```python
from build123d import *

# Parameters (mm, degrees)
F0_R      = 12.7
F1_DEPTH  = 76.2
F3_R      = 17.5641
F4_DEPTH  = 10.16
F6_DEPTH  = 8.636
F7_R      = 12.7
F8_DEPTH  = 76.2
F9_R      = 17.5641
F10_DEPTH = 10.16


with BuildPart() as f1:
    # F0 (on Top) → F1 (new body)
    with BuildSketch(Plane.XY):
        Circle(F0_R)
    extrude(amount=F1_DEPTH)

    # F3 (on offset) → F4 (join)
    with BuildSketch(Plane.XY.offset(74.422)):
        Circle(F3_R)
    extrude(amount=F4_DEPTH)

    # F5 (on Top) → F6 (join)
    with BuildSketch(Plane.XY):
        Polygon((-21.659788, 21.301638), (-21.659788, -20.368967), (60.890212, -20.368967), (60.890212, 0), (60.890212, 21.301638), align=None)
        Polygon((60.890212, 0), (60.890212, -20.368967), (143.440212, -20.368967), (143.440212, 21.301638), (60.890212, 21.301638), align=None)
    extrude(amount=-F6_DEPTH)

    # F7 (on face) → F8 (join)
    with BuildSketch(Plane.XY):
        with Locations((60.890212, 0)):
            Circle(F7_R)
        with Locations((121.774012, 0)):
            Circle(F7_R)
    extrude(amount=F8_DEPTH)

    # F9 (on offset) → F10 (join)
    with BuildSketch(Plane.XY.offset(74.422)):
        with Locations((60.890212, 0)):
            Circle(F9_R)
        with Locations((121.774012, 0)):
            Circle(F9_R)
    extrude(amount=F10_DEPTH)


solid = f1.part
```
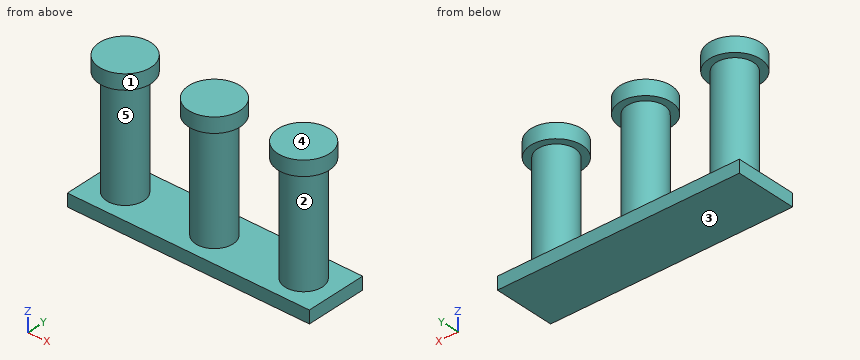
Geometry: final body of the model. Coordinates: model frame, mm. Face numbers are marked on the shaded views. A direction names the side the tool comes from. Round coordinates to 2 decimals unless told otherwise and drop trailing zeros. Write each loop counter-clockwise with the first axis right and the second up, starting at its lowest first coordinate (ties: lowest second). Pieces come first, ordered by that corner, then holes.
Item 1: Section query D-D (y = 0). Return loops of the section in (x, z).
Item 2: Set-up query: the marked faces 1, 2 and 3. Return all of +Z, -Z, +X, -X, +Y, -Y with unobstructed straight access to the full face (end or side cutting, diameter ignored); none if empty.
Item 3: Material intervals for L1, parallel to X at y = 0.5, z = 31; L2, parallel to X at y = 9, z = 17.5; L3, parallel to Z at x = 13, y = -2, sorted ascending.
Item 4: Mould query, pull axis X, two halves, no side actions, for the marked faces 4 and 5. Classes: +X half, -X half, draft (parallel to the pull), parting line (faces both ways), or undercut.
Item 5: Section query B-B (x = 0). Return loops of the section in (y, z).
Item 6: Pin query (flat end, axial travel): P1, Ø12, axis at x = 72.5, z = 40.5, coming from the -Y side; P2, Ø1.5, axis at x = 53, z = 49.5, coming from the +Y side; P3, Ø8, axis at x = 66, z = 64, coming from the -Y side. Return the tip coordinate at first contact, or that it passes through.
Item 7: Section query A-A (y = -16). Return loops of the section in (x, z), plus the area to 3 significant figures.
Item 8: Section query C-C (z = 76.5). Return loops of the section in (x, y), plus the area to 3 significant figures.
Completed:
1. outline: (-21.66, -8.64) - (143.44, -8.64) - (143.44, 0) - (134.47, 0) - (134.47, 74.42) - (139.34, 74.42) - (139.34, 84.58) - (104.21, 84.58) - (104.21, 74.42) - (109.07, 74.42) - (109.07, 0) - (73.59, 0) - (73.59, 74.42) - (78.45, 74.42) - (78.45, 84.58) - (43.33, 84.58) - (43.33, 74.42) - (48.19, 74.42) - (48.19, 0) - (12.7, 0) - (12.7, 74.42) - (17.56, 74.42) - (17.56, 84.58) - (-17.56, 84.58) - (-17.56, 74.42) - (-12.7, 74.42) - (-12.7, 0) - (-21.66, 0) - close
2. face 1: +Z
2. face 2: none
2. face 3: -Z, +X, -X, +Y, -Y
3. L1: x = -12.69 to 12.69, 48.2 to 73.58, 109.08 to 134.46
3. L2: x = -8.96 to 8.96, 51.93 to 69.85, 112.81 to 130.73
3. L3: z = -8.64 to 0, 74.42 to 84.58
4. face 4: draft
4. face 5: undercut
5. outline: (-20.37, -8.64) - (21.3, -8.64) - (21.3, 0) - (12.7, 0) - (12.7, 74.42) - (17.56, 74.42) - (17.56, 84.58) - (-17.56, 84.58) - (-17.56, 74.42) - (-12.7, 74.42) - (-12.7, 0) - (-20.37, 0) - close
6. P1: stops at y = -11.39
6. P2: stops at y = 10.5
6. P3: stops at y = -12.65
7. outline: (-21.66, -8.64) - (143.44, -8.64) - (143.44, 0) - (-21.66, 0) - close; (-7.25, 74.42) - (7.25, 74.42) - (7.25, 84.58) - (-7.25, 84.58) - close; (53.64, 74.42) - (68.14, 74.42) - (68.14, 84.58) - (53.64, 84.58) - close; (114.53, 74.42) - (129.02, 74.42) - (129.02, 84.58) - (114.53, 84.58) - close
7. area: 1,870 mm2
8. outline: circle Ø35.13 at (0, 0); circle Ø35.13 at (60.89, 0); circle Ø35.13 at (121.77, 0)
8. area: 2,910 mm2
